The model under review builds one solid part; all positions refer to its coordinate system, in mm. Coordinates: 2 decimals unless noted, no trailing zeros. Write each loop counter-clockwise with the first axis right and the second up, starting at its lowest first coordinate (ties: lowest second). Pieces come first, ordered by that corner, then holes. Notation, with made-up numbers: (77, -39.5) - (86, -39.5) arc R28 ccw to (86, -18.5) - close; hole circle Ø2 at (56.5, 11.25). An arc over 180 degrees is marked (long way). Use one line per item in the form item = value. Start each with the question number.
Autodesk Inventor part; units mm, degrees
ref_plane "YZ Plane" through (0, 0, 0) normal (1, 0, 0) x (0, 1, 0)
ref_plane "XZ Plane" through (0, 0, 0) normal (0, 1, 0) x (-1, 0, 0)
ref_plane "XY Plane" through (0, 0, 0) normal (0, 0, 1) x (1, 0, 0)
sketch "Sketch1" plane through (0, 0, 0) normal (0, 0, 1) x (1, 0, 0)
  line L0 (0, 35) -> (0, -35)
  line L1 (0, -35) -> (50, -35)
  line L2 (50, 35) -> (0, 35)
  circle A0 centre (50, 0) radius 14
  arc A1 (50, -35) -> (50, 35) centre (50, 0) ccw
  point P0 (0, 0)
  point P1 (0, 0)
  dimension "d11" = 70
  dimension "d12" = 50
  dimension "d14" = 28
extrude "Plate1" add sketch "Sketch1" along normal blind 2
equation "\"d5\" = Thickness"
equation "\"BendReliefWidth\" = Thickness"
equation "\"BendReliefDepth\" = 0.5 * Thickness"
equation "\"CornerReliefSize\" = 4 * Thickness"
equation "\"MinimumRemnant\" = 2 * Thickness"
equation "\"TransitionRadius\" = BendRadius"
equation "\"JacobiRadiusSize\" = BendRadius"
equation "\"GapSize\" = Thickness"
properties part number "AKVA MSC 0512 transverse ring1 4mm 304 8pcs" material "Stainless Steel"
1. Take a section at A-A (y = 0). State the section outline as (x, z) points, plus the area to 3 significant figures.
2. For P1, Ø2, axis at x = 75.5, y = -27, coming from the -Z side, flat-tipped, find the tip position at first contact; note if it passes through.
3. Take a section at D-D (y = -28). State the section outline as (x, z) points.
4. Take a section at B-B (x = 47). State the section outline as (y, z) points, plus the area to 3 significant figures.
5. For L1, parallel to Y at x = 50, z = 0.5; L2, parallel to Y at x = 38, z = 1.8; L3, parallel to X at y = 10, z = 1.5, list the stretches that pass through material, from the lowest coordinate up.
6. Take a section at C-C (z = 1.6). State the section outline as (x, y) points.
7. The part is to be moulded in two halves that separate along X. For faces 1 (the cylindrical face through (36.014, -0.616, 0.986)), 2 (the cylindrical face through (84.99, 0.77, 0.99)), 3 (the flat face through (25, 35, 1)), say which applies: released by +X, released by -X, zero draft, split by the parting line, or undercut.
Returned:
q1.outline = (0, 0) - (36, 0) - (36, 2) - (0, 2) - close; (64, 0) - (85, 0) - (85, 2) - (64, 2) - close
q1.area = 114 mm²
q2.P1 = through
q3.outline = (0, 0) - (71, 0) - (71, 2) - (0, 2) - close
q4.outline = (-35, 0) - (-13.67, 0) - (-13.67, 2) - (-35, 2) - close; (13.67, 0) - (35, 0) - (35, 2) - (13.67, 2) - close
q4.area = 85.3 mm²
q5.L1 = -35 to -14, 14 to 35
q5.L2 = -35 to -7.21, 7.21 to 35
q5.L3 = 0 to 40.2, 59.8 to 83.54
q6.outline = (0, -35) - (50, -35) arc R35 ccw to (50, 35) - (0, 35) - close; hole circle Ø28 at (50, 0)
q7.face_1 = undercut
q7.face_2 = released by +X
q7.face_3 = zero draft
